Could you check a few things on this model? Use its own coordinates, in mm. Face numbers are marked on the shaded views. A direction names the side the tool comes from. Give positions to 0.01 mm unless a question says otherwise; leave off trailing zeros. Loops run counter-clockwise (first coordinate to the right, second up) from the corner with the lowest first, then second, coordinate; pieces in that order, holes last. Notation, with made-up numbers: M 53,-38.5 L 66,-38.5 A18 cw 66,-8.5 Z; hole C -40,-16.5 d3. An arc over 180 degrees is marked long. Answer in a Markdown table with one row per item. Add a question column.
1. If we section it at C-C on x = 2.5: List the corners of the cut face in (y, z) for me, then the cut area to 3 significant figures.
2. Which directions (+Z, -Z, +X, -X, +Y, -Y) give clear straight access to the entire face, cutting with the end or side of a thin tool? Please do the marked faces 1 and 2.
3. I'm going to push flat-ended pins straight in: pin 1 Ø0.5 at (x, z) = (0.5, 1) entering from -Y; pin 2 Ø1 at (x, y) = (11, 2) entering from -Z; pin 3 Ø0.5 at (y, z) = (0, -0.5) entering from -X. Where does each tip first touch, or does it pass through?
4. If we section it at B-B on z = 0: List the corners of the cut face in (x, y) for me (3 decimals).
5. I need wall thicknesses on line 1 along X through (y, z) = (0.25, -2); line 2 along X through (y, z) = (-1, -2.5); line 3 along Y through (x, z) = (9, -0.25). Which ranges of each line are inside material? Lowest first, please. Write a range as from..to.
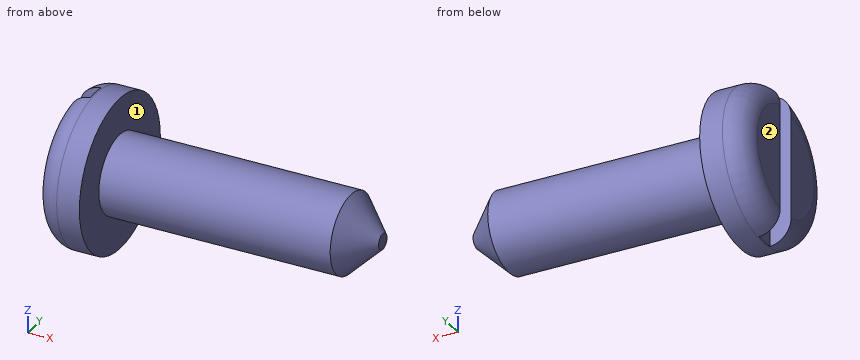
```python
from build123d import *

# Parameters (mm, degrees)
CUT_EXTRUDE1_DEPTH      = 17.145819892
CUT_EXTRUDE1_DEPTH_BACK = 17.145819892
SKETCH2_W               = 1.05
SKETCH2_H               = 1


with BuildPart() as part:
    # Sketch1 → Revolve1 (revolve)
    with BuildSketch(Plane.XY):
        with BuildLine():
            Line((0, 0), (0, 2.625))
            ThreePointArc((0, 2.625), (0.329504871, 3.420495129), (1.125, 3.75))
            Line((1.125, 3.75), (2.25, 3.75))
            Line((2.25, 3.75), (2.25, 1.95))
            Line((2.25, 1.95), (13.69, 1.95))
            Line((13.69, 1.95), (15.25, 0.39))
            Line((15.25, 0.39), (15.25, 0))
            Line((15.25, 0), (0, 0))
        make_face()
    revolve(axis=Axis((15.25, 0, 0), (-1, 0, 0)))

    # Sketch2 → Cut-Extrude1 (cut, two sides: drawn at the far end of the back side and taken through both)
    with BuildSketch(Plane.XY.offset(-CUT_EXTRUDE1_DEPTH_BACK)):
        with Locations((0.525, 0)):
            Rectangle(SKETCH2_W, SKETCH2_H)
    extrude(amount=CUT_EXTRUDE1_DEPTH + CUT_EXTRUDE1_DEPTH_BACK, mode=Mode.SUBTRACT)


solid = part.part
```
Results:
| question | item | result |
|---|---|---|
| 1 | outline | C 0,0 d3.9 |
| 1 | area | 11.9 mm2 |
| 2 | face 1 | +X |
| 2 | face 2 | +Z, -Z, -X, +Y, -Y |
| 3 | pin 1 | y = -3.57 |
| 3 | pin 2 | z = -1.25 |
| 3 | pin 3 | x = 1.05 |
| 4 | outline | M 0,-2.625 A1.125 ccw 1.125,-3.75 L 2.25,-3.75 L 2.25,-1.95 L 13.69,-1.95 L 15.25,-0.39 L 15.25,0.39 L 13.69,1.95 L 2.25,1.95 L 2.25,3.75 L 1.125,3.75 A1.125 ccw 0,2.625 L 0,0.5 L 1.05,0.5 L 1.05,-0.5 L 0,-0.5 Z |
| 5 | line 1 | 1.05..2.25 |
| 5 | line 2 | 0..2.25 |
| 5 | line 3 | -1.93..1.93 |
